```python
from build123d import *

# Parameters (mm, degrees)
F0_R     = 6.35
F1_DEPTH = 19.05


with BuildPart() as f1:
    # F0 (on Front) → F1 (new body)
    with BuildSketch(Plane.XZ):
        with BuildLine():
            ThreePointArc((6.35, -50.8), (4.490128, -46.309872), (0, -44.45))
            ThreePointArc((0, -44.45), (-4.490128, -55.290128), (6.35, -50.8))
        make_face()
        with Locations((50.8, 0)):
            Circle(F0_R)
        with BuildLine():
            Line((26.389365, 23.574162), (24.981764, 24.981764))
            Line((24.981764, 24.981764), (24.948811, 24.948811))
            ThreePointArc((24.948811, 24.948811), (25.661044, 24.253057), (26.389365, 23.574162))
        make_face()
        with BuildLine():
            Line((24.948811, 24.948811), (24.981764, 24.981764))
            Line((24.981764, 24.981764), (23.574162, 26.389365))
            ThreePointArc((23.574162, 26.389365), (24.253057, 25.661044), (24.948811, 24.948811))
        make_face()
        with BuildLine():
            ThreePointArc((26.389365, 23.574162), (25.661044, 24.253057), (24.948811, 24.948811))
            ThreePointArc((24.948811, 24.948811), (24.253057, 25.661044), (23.574162, 26.389365))
            ThreePointArc((23.574162, 26.389365), (16.170482, 37.718625), (12.7, 50.8))
            ThreePointArc((12.7, 50.8), (0, 63.5), (-12.7, 50.8))
            ThreePointArc((-12.7, 50.8), (-25.065625, 25.065625), (-50.8, 12.7))
            ThreePointArc((-50.8, 12.7), (-63.5, 0), (-50.8, -12.7))
            ThreePointArc((-50.8, -12.7), (-36.87956, -16.690866), (-25.065625, -25.065625))
            ThreePointArc((-25.065625, -25.065625), (-16.690866, -36.87956), (-12.7, -50.8))
            ThreePointArc((-12.7, -50.8), (0, -63.5), (12.7, -50.8))
            ThreePointArc((12.7, -50.8), (16.170482, -37.718625), (23.574162, -26.389365))
            ThreePointArc((23.574162, -26.389365), (24.253057, -25.661044), (24.948811, -24.948811))
            ThreePointArc((24.948811, -24.948811), (25.661044, -24.253057), (26.389365, -23.574162))
            ThreePointArc((26.389365, -23.574162), (37.718625, -16.170482), (50.8, -12.7))
            ThreePointArc((50.8, -12.7), (63.432032, 0), (50.8, 12.7))
            ThreePointArc((50.8, 12.7), (37.718625, 16.170482), (26.389365, 23.574162))
        make_face()
        with BuildLine():
            ThreePointArc((6.35, -50.8), (-4.490128, -55.290128), (0, -44.45))
            ThreePointArc((0, -44.45), (4.490128, -46.309872), (6.35, -50.8))
        make_face(mode=Mode.SUBTRACT)
        with Locations((-50.8, 0)):
            Circle(F0_R, mode=Mode.SUBTRACT)
        with BuildLine():
            ThreePointArc((12.7, 0), (8.980256, -8.980256), (0, -12.7))
            ThreePointArc((0, -12.7), (-8.980256, 8.980256), (12.7, 0))
        make_face(mode=Mode.SUBTRACT)
        with Locations((50.8, 0)):
            Circle(F0_R, mode=Mode.SUBTRACT)
        with Locations((0, 50.8)):
            Circle(F0_R, mode=Mode.SUBTRACT)
        with BuildLine():
            Line((24.981764, -24.981764), (26.389365, -23.574162))
            ThreePointArc((26.389365, -23.574162), (25.661044, -24.253057), (24.948811, -24.948811))
            Line((24.948811, -24.948811), (24.981764, -24.981764))
        make_face()
        with BuildLine():
            Line((23.574162, -26.389365), (24.981764, -24.981764))
            Line((24.981764, -24.981764), (24.948811, -24.948811))
            ThreePointArc((24.948811, -24.948811), (24.253057, -25.661044), (23.574162, -26.389365))
        make_face()
    extrude(amount=F1_DEPTH)


solid = f1.part
```
Geometry check sheet. Reference: the model listing, model coordinates, mm. Round coordinates to 2 decimals unless told otherwise and drop trailing zeros. Loops run counter-clockwise (first coordinate to the right, second up) from the corner with the lowest first, then second, coordinate; pieces in that order, holes last. Notation, with made-up numbers: (-39, 58.25) - (-14, 58.25) arc R21 ccw to (-14, 85.25) - close; hole circle Ø2 at (66, 66). An arc over 180 degrees is marked (long way). Write item = value, one per line. Start each with the question number.
1. Section check B-B on z = -49. Enter the section's corners in (x, y), then the cut area to 3 significant figures.
2. Depth check by flat-ended pin: pin 1 (8 mm diameter, centred on y = -6, z = -44.5, fed in from -X); pin 2 (1.5 mm diameter, centred on y = -4, z = -8.5, fed in from -X); pin 3 (1.5 mm diameter, centred on y = -4, z = 12.5, fed in from +X). Enter the tip coordinate at first touch or a pass-through.
3. Section check C-C on x = 43. Enter the section's corners in (y, z), then the cut area to 3 significant figures.
4. Thickness scan on line 1 (X direction, y = -5.5, z = -50.8); line 2 (X direction, y = -0.75, z = 11.5); line 3 (Z direction, x = 54, y = -12.5). Record the ranges inside material, lowest first.
5. Section check A-A on y = -3.5. Enter the section's corners in (x, z).
6. Mould release check, pull along X, two halves, no side actions. Record for faces 1 (the face through (-15, -19.05, 1)), 2 (the face through (-0.8, -9.4, 57.1)), 3 (the face through (37.893, -9.392, 16.093)): released by +X, released by -X, zero draft, split by the parting line, or undercut.
Working result:
q1.outline = (-12.94, -19.05) - (-6.09, -19.05) - (-6.09, 0) - (-12.94, 0) - close; (6.09, -19.05) - (12.92, -19.05) - (12.92, 0) - (6.09, 0) - close
q1.area = 261 mm^2
q2.pin_1 = -15.15
q2.pin_2 = -60.86
q2.pin_3 = 55.55
q3.outline = (-19.05, -14.23) - (0, -14.23) - (0, 14.23) - (-19.05, 14.23) - close
q3.area = 542 mm^2
q4.line_1 = -12.7 to -6.35, 6.35 to 12.7
q4.line_2 = -56.19 to -5.39, 5.39 to 56.12
q4.line_3 = -12.27 to -5.48, 5.48 to 12.27
q5.outline = (-50.8, -12.7) arc R43.12 cw to (-25.07, -25.07) arc R43.12 cw to (-12.7, -50.8) arc R12.7 ccw to (12.7, -50.8) arc R42.54 cw to (23.57, -26.39) - (24.98, -24.98) - (26.39, -23.57) arc R42.54 cw to (50.8, -12.7) arc R12.7 ccw to (50.8, 12.7) arc R42.54 cw to (26.39, 23.57) - (24.98, 24.98) - (23.57, 26.39) arc R42.54 cw to (12.7, 50.8) arc R12.7 ccw to (-12.7, 50.8) arc R43.12 cw to (-50.8, 12.7) arc R12.7 ccw to start; hole circle Ø12.7 at (-50.8, 0); hole circle Ø25.4 at (0, 0); hole circle Ø12.7 at (0, -50.8); hole circle Ø12.7 at (0, 50.8); hole circle Ø12.7 at (50.8, 0)
q6.face_1 = zero draft
q6.face_2 = undercut
q6.face_3 = released by +X
